Check sheet for the modelled part. Datum: model origin and axes. Units: mm. A direction names the side the tool comes from. Coordinates: 2 decimals unless noted, no trailing zeros. Loops run counter-clockwise (first coordinate to the right, second up) from the corner with the lowest first, then second, coordinate; pieces in that order, holes last. Notation, with made-up numbers: M -13,18.5 L 13,18.5 A31 cw 13,46.5 Z; hole C 58.25,60 d11. An arc over 180 degrees is marked long. Use CSV: the item, a comma, the result in double quotes. Start each with the question number.
(1) Scan lines: line 1 (Z direction, x = 16, y = 12.25); line 2 (X direction, y = 3.75, z = 4.75); line 3 (X direction, y = 6.25, z = 0.4). Record each from-to range of solid material in increasing order.
(2) Draft check along Y on faces 1 (the flat face through (16, 7, 3)), 2 (the flat face through (9, 14, 3)), 3 (the flat face through (9, 0, 3)). Enter one of: pulls with the +Y half, pulls with the -Y half, needs draft (parallel to the pull), parting line crosses it, or undercut.
(3) Go/stop test with a flat-tipped pin: pin 1 Ø0.6 at (y, z) = (5, 4.5) entering from +X. Record where the tip stops, or that it passes through.
(4) Section check A-A on z = 4.45. Record the cut outline in (x, y), and give its area (3 significant figures).
(5) Set-up check for faces 4 (the flat face through (9, 7, 0)), 5 (the flat face through (15, 7, 5)): record each of +Z, -Z, +X, -X, +Y, -Y from which the full face is reachable in a straight line by a thin tool's end or side.
(6) Section check B-B on y = 10.5. Record the cut outline in (x, z), and give its area (3 significant figures).
Autodesk Inventor part; units mm, degrees
ref_plane "YZ Plane" through (0, 0, 0) normal (1, 0, 0) x (0, 1, 0)
ref_plane "XZ Plane" through (0, 0, 0) normal (0, 1, 0) x (-1, 0, 0)
ref_plane "XY Plane" through (0, 0, 0) normal (0, 0, 1) x (1, 0, 0)
sketch "Sketch1" plane through (0, 0, 0) normal (0, 0, 1) x (1, 0, 0)
  line L0 (0, 0) -> (18, 0)
  line L1 (18, 0) -> (18, 14)
  line L2 (18, 14) -> (0, 14)
  line L3 (0, 14) -> (0, 0)
  dimension "d0" = 18
  dimension "d1" = 14
extrude "Extrusion1" add sketch "Sketch1" along normal blind 6
sketch "Sketch2" plane through (0, 0, 0) normal (0, -1, 0) x (1, 0, 0)
  line L0 (18, 6) -> (15, 6)
  line L1 (15, 6) -> (15, 3)
  line L2 (15, 3) -> (18, 3)
  line L3 (18, 3) -> (18, 6)
  point P0 (0, 0)
  dimension "d5" = 3
  dimension "d6" = 3
extrude "Extrusion2" cut sketch "Sketch2" against normal up to next
fillet "Fillet1" radius 0.5 18 edges at (0, 7, 0) (0, 0, 3) (0, 7, 6) (0, 14, 3) (9, 14, 0) (7.5, 14, 6) (18, 14, 1.5) (18, 7, 0) (18, 0, 1.5) (9, 0, 0) (7.5, 0, 6) (15, 7, 3) (15, 7, 6) (15, 0, 4.5) (16.5, 0, 3) (16.5, 14, 3) (18, 7, 3) (15, 14, 4.5)
properties part number "battery"
Outcome:
1,line 1,"z = 0 to 3"
1,line 2,"x = 0 to 15"
1,line 3,"x = 0.01 to 17.99"
2,face 1,"needs draft"
2,face 2,"pulls with the +Y half"
2,face 3,"pulls with the -Y half"
3,pin 1,"stops at x = 15"
4,outline,"M 0,0.5 A0.5 ccw 0.5,0 L 14.5,0 A0.5 ccw 15,0.5 L 15,13.5 A0.5 ccw 14.5,14 L 0.5,14 A0.5 ccw 0,13.5 Z"
4,area,"210 mm²"
5,face 4,"-Z, +X, -X, +Y, -Y"
5,face 5,"+Z, +X, +Y, -Y"
6,outline,"M 0,0.5 A0.5 ccw 0.5,0 L 17.5,0 A0.5 ccw 18,0.5 L 18,2.5 A0.5 ccw 17.5,3 L 15.5,3 A0.5 cw 15,3.5 L 15,5.5 A0.5 ccw 14.5,6 L 0.5,6 A0.5 ccw 0,5.5 Z"
6,area,"98.8 mm²"
